Source: CAD feature listing. Evaluate the final solid. Frame: model axes, mm. A direction names the side the tool comes from. Round coordinates to 2 decimals unless told otherwise and drop trailing zeros. Loops run counter-clockwise (first coordinate to the right, second up) from the corner with the lowest first, then second, coordinate; pieces in that order, holes last.
Item 1: Pull-direction query (Y, two-part tool) for faces 1 (the flat face through (-16.17, 131.38, 6.41)), 2 (the cylindrical face through (-2.225, 87.362, 9.056)), 3 (the cylindrical face through (-1.7, -22.62, 9.06)), 4 (the flat face through (-7.3, 54.6, 13)); classes: released by +Y, released by -Y, zero draft, split by the parting line, or undercut.
Item 2: Section query C-C on y = 10.5. Return loops of the section in (x, z).
Item 3: First-contact query: P1, Ø6, axis at y = 61, z = 9, coming from the +X side; P2, Ø5, axis at y = 126.5, z = 11.5, coming from the +X side; P3, Ø1.5, axis at y = 130, z = 5.5, coming from the -X side. Flat tips, straight axial feed; report the tip coordinate or a pass-through.
Item 4: Section query D-D on y = -28. Return loops of the section in (x, z), then the cut area to 3 significant figures.
Item 5: Ray query, L1, parallel to Y at x = -4, z = 7; L2, parallel to Z at x = 0.5, y = -15; L3, parallel to X at y = -3, z = 8.5. Return the intervals inside material, ascending.
Item 6: Section query A-A on z = 8.25. Return loops of the section in (x, y).
Item 7: Access query for faces 5 (the flat face through (-2, 33, 5)), 6 (the flat face through (-11.115, 36, 6)), 7 (the cylindrical face through (-10.741, 151.095, 6.409)). Directions: +Z, -Z, +X, -X, +Y, -Y. A direction counts if a zero-diameter tool reaches every point of the face in a straight line with its end or side. Return the directions, or none.
Item 8: Section query B-B on y = 60. Return loops of the section in (x, z).
```python
from build123d import *

# Parameters (mm, degrees)
SKETCH1_R      = 2.5
EXTRUDE1_DEPTH = 13
EXTRUDE2_DEPTH = 8


with BuildPart() as part:
    # Sketch1 → Extrude1 (new body)
    with BuildSketch(Plane.XY):
        with BuildLine():
            Line((-11.114615619, 113.277430864), (-11.114615619, -42.636308558))
            ThreePointArc((-11.114615619, -42.636308558), (-2.114615619, -51.636308558), (6.885384381, -42.636308558))
            Line((6.885384381, -42.636308558), (6.565118116, 114.072785693))
            ThreePointArc((6.565118116, 114.072785693), (6.384581051, 115.236243879), (6.053710916, 116.36617907))
            Line((6.053710916, 116.36617907), (-3.084934036, 148.987312466))
            ThreePointArc((-3.084934036, 148.987312466), (-12.084934036, 157.987312466), (-21.084934036, 148.987312466))
            Line((-21.084934036, 148.987312466), (-11.114615619, 113.277430864))
        make_face()
        with Locations((-2.399669149, 113.277430864)):
            Circle(SKETCH1_R, mode=Mode.SUBTRACT)
        with Locations((-2.114615619, -42.636308558)):
            Circle(SKETCH1_R, mode=Mode.SUBTRACT)
        with Locations((-12.084934036, 148.987312466)):
            Circle(SKETCH1_R, mode=Mode.SUBTRACT)
    extrude(amount=EXTRUDE1_DEPTH)

    # Sketch2 → Extrude2 (cut)
    with BuildSketch(Plane.XY.offset(13)):
        with BuildLine():
            Line((2.885384381, 82.363691442), (2.828618024, -16.885015572))
            ThreePointArc((2.828618024, -16.885015572), (-1.817326792, -22.627462668), (-7.112080712, -17.477114833))
            Line((-7.112080712, -17.477114833), (-7.114615619, 82.363691442))
            ThreePointArc((-7.114615619, 82.363691442), (-2.114615619, 87.363691442), (2.885384381, 82.363691442))
        make_face()
    extrude(amount=-EXTRUDE2_DEPTH, mode=Mode.SUBTRACT)


solid = part.part
```
Data:
1. face 1: released by -Y
1. face 2: undercut
1. face 3: undercut
1. face 4: zero draft
2. outline: (-11.11, 0) - (6.78, 0) - (6.78, 13) - (2.84, 13) - (2.84, 5) - (-7.11, 5) - (-7.11, 13) - (-11.11, 13) - close
3. P1: stops at x = 6.68
3. P2: stops at x = 3.92
3. P3: stops at x = -15.99
4. outline: (-11.11, 0) - (6.86, 0) - (6.86, 13) - (-11.11, 13) - close
4. area: 234 mm2
5. L1: y = -51.44 to -44.28, -40.99 to -22.27, 86.99 to 111.36, 115.2 to 152.94
5. L2: z = 0 to 5
5. L3: x = -11.11 to -7.11, 2.84 to 6.8
6. outline: (-21.08, 148.99) - (-11.11, 113.28) - (-11.11, -42.64) arc R9 ccw to (6.89, -42.64) - (6.57, 114.07) arc R9 ccw to (6.05, 116.37) - (-3.08, 148.99) arc R9 ccw to start; hole circle Ø5 at (-12.08, 148.99); hole (-7.11, -17.48) arc R5 ccw (long way) to (2.83, -16.89) - (2.89, 82.36) arc R5 ccw to (-7.11, 82.36) - close; hole circle Ø5 at (-2.4, 113.28); hole circle Ø5 at (-2.11, -42.64)
7. face 5: +Z
7. face 6: +Z, -Z, -X, -Y
7. face 7: +Z, -Z
8. outline: (-11.11, 0) - (6.68, 0) - (6.68, 13) - (2.87, 13) - (2.87, 5) - (-7.11, 5) - (-7.11, 13) - (-11.11, 13) - close
